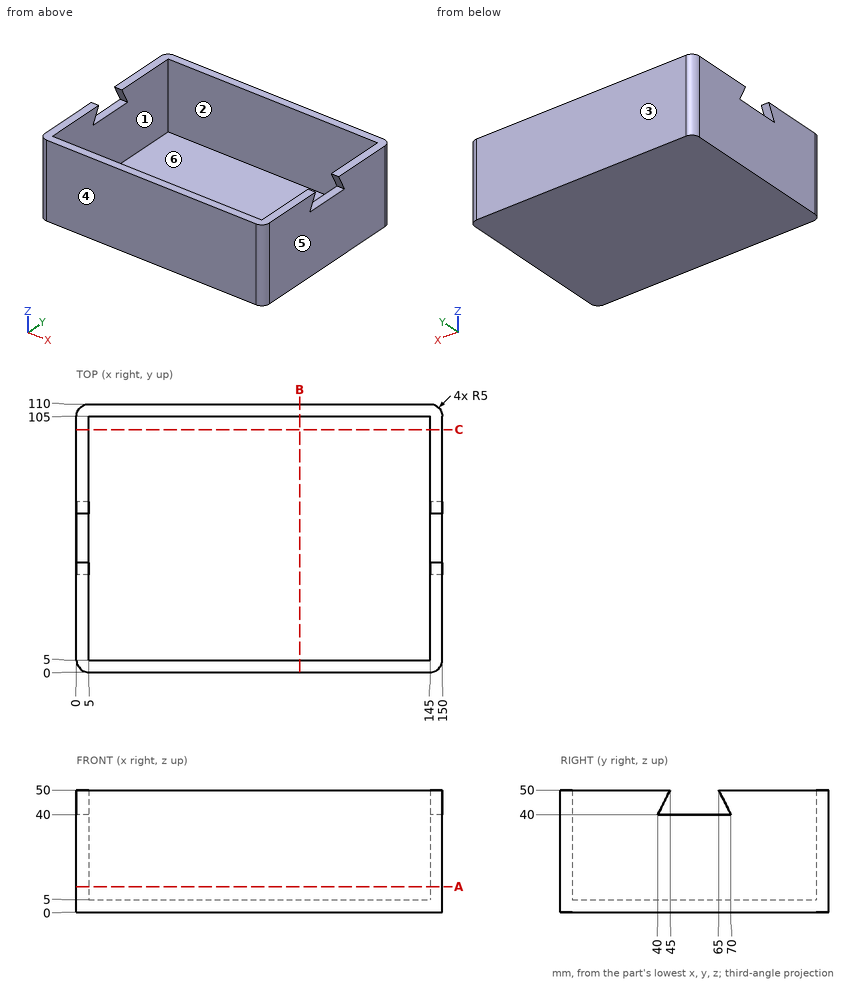
The drawing under review shows one solid part. Ordinate dimensions are in mm from its lowest x, y, z. A direction names the side the tool comes from. Give positions to 0.01 mm unless a question says otherwise; leave off trailing zeros. Write each loop counter-clockwise with the first axis right and the second up, starting at its lowest first coordinate (ties: lowest second). Pieces come first, ordered by that corner, then holes.
1. Wall thickness on L1, parallel to Y at x = 89, z = 26; L2, parallel to X at y = 93.5, z = 8; L3, parallel to Z at x = 113, y = 9: over which ranges is each line inside the solid? List them lowest first.
2. Draft analysis for pull direction Y (two halves, no side actions). For the marked faces 1, 2, 3 and 4, state which applies: +Y half, -Y half, draft (parallel to the pull), parting line (faces both ways), or undercut.
3. Add section C-C, the plane y = 99.5. Write out the cut boundary in (x, z), plus the area to 3 significant figures.
4. Tool access review of the marked faces 5 and 6: name each direction out of +Z, -Z, +X, -X, +Y, -Y from which nothing blocks a thin tool from reaching the whole face with its end or side.
5. Add section B-B, the plane x = 91.5. Write out the cut boundary in (y, z).
6. Add section A-A, the plane z = 10.5. Write out the cut boundary in (x, y), plus the area to 3 significant figures.
7. For P1, Ø5.5, axis at x = 3.5, y = 58.5, coming from the +Z side; P2, Ø2, axis at x = 130, z = 24, coming from the -Y side; P3, Ø3, axis at x = 83.5, y = 79.5, coming from the +Z side, all flat-tipped, find the tip position at first contact; note any pin that passes through.
Worked answers:
1. L1: y = 0 to 5, 105 to 110
1. L2: x = 0 to 5, 145 to 150
1. L3: z = 0 to 5
2. face 1: undercut
2. face 2: undercut
2. face 3: +Y half
2. face 4: -Y half
3. outline: (0, 0) - (150, 0) - (150, 50) - (145, 50) - (145, 5) - (5, 5) - (5, 50) - (0, 50) - close
3. area: 1,200 mm2
4. face 5: +Z, -Z, +X, +Y, -Y
4. face 6: +Z
5. outline: (0, 0) - (110, 0) - (110, 50) - (105, 50) - (105, 5) - (5, 5) - (5, 50) - (0, 50) - close
6. outline: (0, 5) arc R5 ccw to (5, 0) - (145, 0) arc R5 ccw to (150, 5) - (150, 105) arc R5 ccw to (145, 110) - (5, 110) arc R5 ccw to (0, 105) - close; hole (5, 5) - (145, 5) - (145, 105) - (5, 105) - close
6. area: 2,480 mm2
7. P1: stops at z = 40
7. P2: stops at y = 0
7. P3: stops at z = 5
